Geometry: final body of the model. Coordinates: model frame, mm. A direction names the side the tool comes from. Coordinates: 2 decimals unless noted, no trailing zeros. Order: outer loops, then holes, each group sorted by start corner. A loop starts at its lowest first (then second) coordinate and runs counter-clockwise, first axis right, second up. Notation, with made-up numbers: M -9,-4 L -2,-4 A26 cw -2,32 Z; hole C 69.5,10.5 d7. An arc over 180 degrees is marked long. Use CSV: the item, a comma, the result in double quotes. Start each with the question number.
1. Section query A-A on y = -0.5. Return the cut outline in (x, z) (1 decimal).
2. Pull-direction query (X, two-part tool) for faces 3 (the cylindrical face through (0.751, 8.742, -110.015)), 4 (the flat face through (-9, 0, -161.925)); classes: pulls with the +X half, pulls with the -X half, needs draft (parallel to the pull), parting line crosses it, or undercut.
3. Set-up query: faces 1 (the cylindrical face through (0.1, -8.7, -22.5)), 2 (the flat face through (-7.938, 0, 2)). Return all of +Z, -Z, +X, -X, +Y, -Y with unobstructed straight access to the full face (end or side cutting, diameter ignored); none if empty.
4. Section query B-B on z = 18.5. Return the cut outline in (x, y) (1 decimal).
5. First-contact query: P1, Ø8, axis at x = 0, z = -40, coming from the -Y side (3 decimals); P2, Ø3, axis at x = 0, z = 112.4, coming from the +Y side. Flat tips, straight axial feed; report the tip coordinate or a pass-through.
6. Material intervals for line 1 (X direction, y = -7.25, z = -97.5) (1 decimal); line 2 (X direction, y = 8.6, z = -20) (3 decimals), sorted ascending.
from build123d import *

# Parameters (mm, degrees)
SKETCH1_W           = 19.05
SKETCH1_H           = 19.05
SKETCH1_W_2         = 15.875
SKETCH1_H_2         = 15.875
BOSS_EXTRUDE1_DEPTH = 161.925
SKETCH2_R           = 2.5
CUT_EXTRUDE1_DEPTH  = 30
SKETCH3_R           = 2.5
CUT_EXTRUDE2_DEPTH  = 30


with BuildPart() as part:
    # Sketch1 → Boss-Extrude1 (new, symmetric)
    with BuildSketch(Plane.XY):
        Rectangle(SKETCH1_W, SKETCH1_H)
        Rectangle(SKETCH1_W_2, SKETCH1_H_2, mode=Mode.SUBTRACT)
    extrude(amount=BOSS_EXTRUDE1_DEPTH, both=True)

    # Sketch2 → Cut-Extrude1 (cut)
    with BuildSketch(Plane(origin=(-206.375, 13.525, 0), x_dir=(0, 0, -1), z_dir=(0, 1, 0))):
        with Locations(Location((152.4, -206.375, 0), (0, 0, 180))):
            Circle(SKETCH2_R)
        with Locations(Location((132.4, -206.375, 0), (0, 0, 180))):
            Circle(SKETCH2_R)
        with Locations(Location((112.4, -206.375, 0), (0, 0, 180))):
            Circle(SKETCH2_R)
    cut_extrude1 = extrude(amount=-CUT_EXTRUDE1_DEPTH, mode=Mode.SUBTRACT)

    # Mirror1: Cut-Extrude1 across Front Plane
    add(cut_extrude1.mirror(Plane.XY), mode=Mode.SUBTRACT)

    # Sketch3 → Cut-Extrude2 (cut)
    with BuildSketch(Plane(origin=(-206.375, 13.525, 0), x_dir=(0, 0, -1), z_dir=(0, 1, 0))):
        with Locations(Location((0, -206.375, 0), (0, 0, 180))):
            Circle(SKETCH3_R)
        with Locations(Location((20, -206.375, 0), (0, 0, 180))):
            Circle(SKETCH3_R)
        with Locations(Location((40, -206.375, 0), (0, 0, 180))):
            Circle(SKETCH3_R)
    extrude(amount=-CUT_EXTRUDE2_DEPTH, mode=Mode.SUBTRACT)


solid = part.part
Results list:
1,outline,"M -9.5,-161.9 L -7.9,-161.9 L -7.9,161.9 L -9.5,161.9 Z; M 7.9,-161.9 L 9.5,-161.9 L 9.5,161.9 L 7.9,161.9 Z"
2,face 3,"undercut"
2,face 4,"needs draft"
3,face 1,"+Y, -Y"
3,face 2,"+Z, -Z"
4,outline,"M -9.5,-9.5 L 9.5,-9.5 L 9.5,9.5 L -9.5,9.5 Z; hole M -7.9,-7.9 L 7.9,-7.9 L 7.9,7.9 L -7.9,7.9 Z"
5,P1,"stops at y = -9.525"
5,P2,"passes through"
6,line 1,"x = -9.5 to -7.9, 7.9 to 9.5"
6,line 2,"x = -9.525 to -2.5, 2.5 to 9.525"
